Design review of the part built by this model. Coordinates are the model's own, in mm. Face numbers are marked on the shaded views. Give positions to 0.01 mm unless a question says otherwise; leave off trailing zeros. Loops run counter-clockwise (first coordinate to the right, second up) from the corner with the lowest first, then second, coordinate; pieces in that order, holes last.
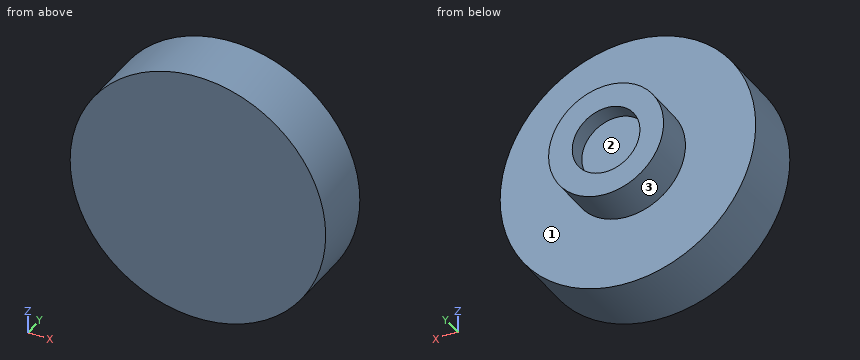
from build123d import *

# Parameters (mm, degrees)
SKETCH1_R           = 4.5
SKETCH1_R_2         = 2.65
BOSS_EXTRUDE1_DEPTH = 3.8
SKETCH2_R           = 2.65
BOSS_EXTRUDE2_DEPTH = 1.8
SKETCH3_R           = 10
BOSS_EXTRUDE3_DEPTH = 5
SKETCH4_R           = 6.809110127
CUT_EXTRUDE1_DEPTH  = 0.6


with BuildPart() as part:
    # Sketch1 → Boss-Extrude1 (new body)
    with BuildSketch(Plane(origin=(0, 0, 0), x_dir=(1, 0, 0), z_dir=(0, 1, 0))):
        Circle(SKETCH1_R)
        Circle(SKETCH1_R_2, mode=Mode.SUBTRACT)
    extrude(amount=BOSS_EXTRUDE1_DEPTH)

    # Sketch2 → Boss-Extrude2 (add)
    with BuildSketch(Plane.XZ):
        Circle(SKETCH2_R)
    extrude(amount=-BOSS_EXTRUDE2_DEPTH)

    # Sketch3 → Boss-Extrude3 (add)
    with BuildSketch(Plane.XZ):
        Circle(SKETCH3_R)
    extrude(amount=BOSS_EXTRUDE3_DEPTH)

    # Sketch4 → Cut-Extrude1 (cut)
    with BuildSketch(Plane(origin=(0, 3.8, 0), x_dir=(1, 0, 0), z_dir=(0, 1, 0))):
        Circle(SKETCH4_R)
    extrude(amount=-CUT_EXTRUDE1_DEPTH, mode=Mode.SUBTRACT)


solid = part.part
Q1. Take a section at C-C (y = 2.5). Give the boundary of the cut face in (x, z), plus the area to 3 significant figures.
Results:
outline: circle Ø9 at (0, 0); hole circle Ø5.3 at (0, 0)
area: 41.6 mm2
Q2. Take a section at A-A (x = 0). Give the boundary of the cut face in (y, z).
Results:
outline: (-5, -10) - (0, -10) - (0, -4.5) - (3.2, -4.5) - (3.2, -2.65) - (1.8, -2.65) - (1.8, 2.65) - (3.2, 2.65) - (3.2, 4.5) - (0, 4.5) - (0, 10) - (-5, 10) - close
Q3. Take a section at D-D (y = -2). Give the boundary of the cut face in (x, z), plus the area to 3 significant figures.
Results:
outline: circle Ø20 at (0, 0)
area: 314 mm2
Q4. Take a section at B-B (z = 0). Give the boundary of the cut face in (x, y), plus the area to 3 significant figures.
Results:
outline: (-10, -5) - (10, -5) - (10, 0) - (4.5, 0) - (4.5, 3.2) - (2.65, 3.2) - (2.65, 1.8) - (-2.65, 1.8) - (-2.65, 3.2) - (-4.5, 3.2) - (-4.5, 0) - (-10, 0) - close
area: 121 mm2
Q5. Draft analysis for pull direction X (two halves, no side actions). For the marked faces 1, 2 and 3, state which applies: pulls with the +X half, pulls with the -X half, needs draft (parallel to the pull), parting line crosses it, or undercut.
Results:
face 1: needs draft
face 2: undercut
face 3: parting line crosses it
Q6. Wall thickness on line 1 (Z direction, x = 0, y = 2.6); line 2 (Y direction, x = 5, z = -3); line 3 (Y direction, x = 0.25, z = -1.5): over which ranges is each line inside the solid? List them lowest first.
Results:
line 1: z = -4.5 to -2.65, 2.65 to 4.5
line 2: y = -5 to 0
line 3: y = -5 to 1.8
Q7. Insertion check: pin 1 (2 mm diameter, centred on y = -4, z = -4.5, fed in from -X); pin 2 (3 mm diameter, centred on y = -0.5, z = 6, fed in from -X). Each pin has a flat end and moves straight along its axis. Give the tip position at first contact, or say it passes through.
Results:
pin 1: stops at x = -9.37
pin 2: stops at x = -8.93
